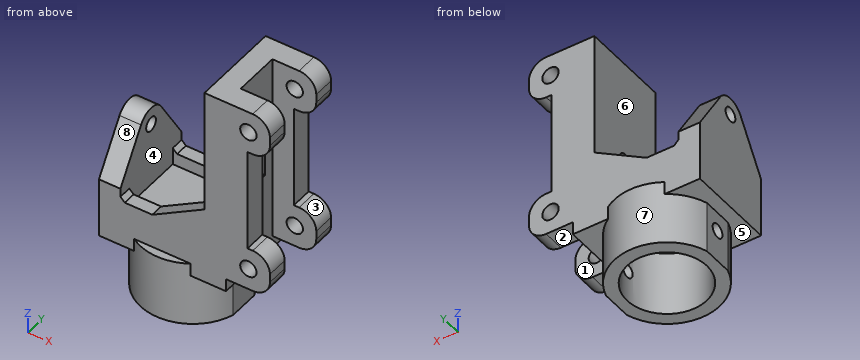
from build123d import *

# Parameters (mm, degrees)
SKETCH_1_R               = 6.325
EXTRUDE_1_DEPTH          = 15
SKETCH_2_W               = 29.5
SKETCH_2_H               = 20.7
EXTRUDE_2_DEPTH          = 5
SKETCH_3_W               = 39
SKETCH_3_H               = 20.7
SKETCH_3_R               = 1.65
EXTRUDE_3_DEPTH          = 5
SKETCH_4_W               = 10
SKETCH_4_H               = 5
EXTRUDE_4_DEPTH          = 10.2
SKETCH_5_R               = 1.9
CUT_EXTRUDE_1_DEPTH      = 21.7
FILLET_1_R               = 4
SKETCH_8_W               = 24
SKETCH_8_H               = 5
EXTRUDE_6_DEPTH          = 5
SKETCH_9_R               = 1.65
EXTRUDE_7_DEPTH          = 5
EXTRUDE_5_DEPTH          = 3
CHAMFER_2_SIZE           = 1
SKETCH_10_W              = 6.3
SKETCH_10_H              = 5.8
CUT_EXTRUDE_2_DEPTH      = 2.5
SKETCH_11_R              = 1.65
CUT_EXTRUDE_3_DEPTH      = 25.95
CUT_EXTRUDE_3_DEPTH_BACK = 15.75
CHAMFER_3_SIZE           = 1
CUT_EXTRUDE_4_DEPTH      = 1
CUT_EXTRUDE_4_DEPTH_BACK = 21.7
SKETCH_13_R              = 12.25
SKETCH_13_R_2            = 9.25
EXTRUDE_8_DEPTH          = 15
SKETCH_14_R              = 1.65
CUT_EXTRUDE_5_DEPTH      = 25.95
CUT_EXTRUDE_5_DEPTH_BACK = 15.75
SKETCH_15_W              = 4.137033229
SKETCH_15_H              = 7
CUT_EXTRUDE_6_DEPTH      = 15
EXTRUDE_9_DEPTH          = 3


with BuildPart() as part:
    # ｽｹｯﾁ1 → ﾎﾞｽ - 押し出し1 (new body)
    with BuildSketch(Plane.XY):
        Circle(SKETCH_1_R)
    extrude(amount=-EXTRUDE_1_DEPTH)

    # ｽｹｯﾁ2 → ﾎﾞｽ - 押し出し2 (add)
    with BuildSketch(Plane.XY):
        Rectangle(SKETCH_2_W, SKETCH_2_H)
    extrude(amount=EXTRUDE_2_DEPTH)

    # ｽｹｯﾁ3 → ﾎﾞｽ - 押し出し3 (add)
    with BuildSketch(Plane(origin=(14.75, 0, 0), x_dir=(0, 0, -1), z_dir=(1, 0, 0))):
        with Locations((-24.5, 0)):
            Rectangle(SKETCH_3_W, SKETCH_3_H)
        with Locations((-20, 0)):
            Circle(SKETCH_3_R, mode=Mode.SUBTRACT)
    extrude(amount=-EXTRUDE_3_DEPTH)

    # ｽｹｯﾁ4 → ﾎﾞｽ - 押し出し4 (add)
    with BuildSketch(Plane(origin=(14.75, 0, 0), x_dir=(0, 0, -1), z_dir=(1, 0, 0))):
        with Locations((-5, 7.85)):
            Rectangle(SKETCH_4_W, SKETCH_4_H)
        with Locations((-5, -7.85)):
            Rectangle(SKETCH_4_W, SKETCH_4_H)
        with Locations((-39, 7.85)):
            Rectangle(SKETCH_4_W, SKETCH_4_H)
        with Locations((-39, -7.85)):
            Rectangle(SKETCH_4_W, SKETCH_4_H)
    extrude(amount=EXTRUDE_4_DEPTH)

    # ｽｹｯﾁ5 → ｶｯﾄ - 押し出し1 (cut, through all)
    with BuildSketch(Plane.XZ.offset(10.35)):
        with Locations((19.95, 5)):
            Circle(SKETCH_5_R)
        with Locations((19.95, 39)):
            Circle(SKETCH_5_R)
    extrude(amount=-CUT_EXTRUDE_1_DEPTH, mode=Mode.SUBTRACT)

    # ﾌｨﾚｯﾄ1
    fillet_1_edges = [part.edges().sort_by_distance(p)[0] for p in [
        (24.95, 7.85, 0),
        (24.95, 7.85, 10),
        (24.95, -7.85, 0),
        (24.95, -7.85, 10),
        (24.95, -7.85, 44),
        (24.95, -7.85, 34),
        (24.95, 7.85, 44),
        (24.95, 7.85, 34),
    ]]
    fillet(fillet_1_edges, radius=FILLET_1_R)

    # ｽｹｯﾁ8 → ﾎﾞｽ - 押し出し6 (add)
    with BuildSketch(Plane(origin=(14.75, 0, 0), x_dir=(0, 0, -1), z_dir=(1, 0, 0))):
        with Locations((-22, 7.85)):
            Rectangle(SKETCH_8_W, SKETCH_8_H)
        with Locations((-22, -7.85)):
            Rectangle(SKETCH_8_W, SKETCH_8_H)
    extrude(amount=EXTRUDE_6_DEPTH)

    # ｽｹｯﾁ9 → ﾎﾞｽ - 押し出し7 (add)
    with BuildSketch(Plane.ZY.offset(14.75)):
        with BuildLine():
            Line((5, 10.35), (11, 10.35))
            Line((11, 10.35), (22.121751649, 3.390895153))
            ThreePointArc((22.121751649, 3.390895153), (24, 0), (22.121751649, -3.390895153))
            Line((22.121751649, -3.390895153), (11, -10.35))
            Line((11, -10.35), (5, -10.35))
            Line((5, -10.35), (5, 10.35))
        make_face()
        with Locations((20, 0)):
            Circle(SKETCH_9_R, mode=Mode.SUBTRACT)
    extrude(amount=-EXTRUDE_7_DEPTH)

    # ｽｹｯﾁ6 → ﾎﾞｽ - 押し出し5 (add)
    with BuildSketch(Plane.XZ.offset(10.35)):
        Polygon((-9.75, 5), (9.75, 5), (9.75, 15), (-2.374355653, 8), (-9.75, 8), align=None)
    extrude_5 = extrude(amount=-EXTRUDE_5_DEPTH)

    # ﾐﾗｰ1: ﾎﾞｽ - 押し出し5 across plane
    add(extrude_5.mirror(Plane.ZX))

    # 面取り2
    chamfer_2_edges = [part.edges().sort_by_distance(p)[0] for p in [
        (-9.75, -8.85, 8),
        (-9.75, 8.85, 8),
    ]]
    chamfer(chamfer_2_edges, length=CHAMFER_2_SIZE)

    # ｽｹｯﾁ10 → ｶｯﾄ - 押し出し2 (cut)
    with BuildSketch(Plane(origin=(14.75, 0, 0), x_dir=(0, 0, -1), z_dir=(1, 0, 0))):
        with Locations((-20, 0)):
            Rectangle(SKETCH_10_W, SKETCH_10_H)
    extrude(amount=-CUT_EXTRUDE_2_DEPTH, mode=Mode.SUBTRACT)

    # ｽｹｯﾁ11 → ｶｯﾄ - 押し出し3 (cut, two sides)
    with BuildSketch(Plane(origin=(0, 0, 0), x_dir=(0, 0, -1), z_dir=(1, 0, 0))) as cut_extrude_3_sk:
        with Locations((7.5, 0)):
            Circle(SKETCH_11_R)
    extrude(amount=CUT_EXTRUDE_3_DEPTH, mode=Mode.SUBTRACT)
    extrude(cut_extrude_3_sk.sketch, amount=-CUT_EXTRUDE_3_DEPTH_BACK, mode=Mode.SUBTRACT)

    # 面取り3
    chamfer_3_edges = [part.edges().sort_by_distance(p)[0] for p in [
        (-6.325, 0, -15),
    ]]
    chamfer(chamfer_3_edges, length=CHAMFER_3_SIZE)

    # ｽｹｯﾁ12 → ｶｯﾄ - 押し出し4 (cut, two sides)
    with BuildSketch(Plane(origin=(0, 10.35, 0), x_dir=(1, 0, 0), z_dir=(0, 1, 0))) as cut_extrude_4_sk:
        Polygon((-157.887970151, 0), (-20.856584832, 0), (30.621949215, 0), (167.653334534, 0), (167.653334534, 274.062770638), (-157.887970151, 274.062770638), align=None)
    extrude(amount=CUT_EXTRUDE_4_DEPTH, mode=Mode.SUBTRACT)
    extrude(cut_extrude_4_sk.sketch, amount=-CUT_EXTRUDE_4_DEPTH_BACK, mode=Mode.SUBTRACT)

    # ｽｹｯﾁ13 → ﾎﾞｽ - 押し出し8 (add)
    with BuildSketch(Plane(origin=(0, 0, 0), x_dir=(-1, 0, 0), z_dir=(0, 0, -1))):
        Circle(SKETCH_13_R)
        Circle(SKETCH_13_R_2, mode=Mode.SUBTRACT)
    extrude(amount=EXTRUDE_8_DEPTH)

    # ｽｹｯﾁ14 → ｶｯﾄ - 押し出し5 (cut, two sides)
    with BuildSketch(Plane(origin=(0, 0, 0), x_dir=(0, 0, -1), z_dir=(1, 0, 0))) as cut_extrude_5_sk:
        with Locations((7.5, 0)):
            Circle(SKETCH_14_R)
    extrude(amount=CUT_EXTRUDE_5_DEPTH, mode=Mode.SUBTRACT)
    extrude(cut_extrude_5_sk.sketch, amount=-CUT_EXTRUDE_5_DEPTH_BACK, mode=Mode.SUBTRACT)

    # ｽｹｯﾁ15 → ｶｯﾄ - 押し出し6 (cut)
    with BuildSketch(Plane(origin=(0, 0, -15), x_dir=(-1, 0, 0), z_dir=(0, 0, -1))):
        with Locations((-13.807873497, 0)):
            Rectangle(SKETCH_15_W, SKETCH_15_H)
        with Locations((13.807873497, 0)):
            Rectangle(SKETCH_15_W, SKETCH_15_H)
    extrude(amount=-CUT_EXTRUDE_6_DEPTH, mode=Mode.SUBTRACT)

    # ｽｹｯﾁ16 → ﾎﾞｽ - 押し出し9 (add)
    with BuildSketch(Plane(origin=(0, 0, 0), x_dir=(-1, 0, 0), z_dir=(0, 0, -1))):
        with BuildLine():
            Line((-11.739356882, 3.5), (-11.739356882, -3.5))
            ThreePointArc((-11.739356882, -3.5), (-9.766367935, -7.394630306), (-6.55286197, -10.35))
            Line((-6.55286197, -10.35), (-14.75, -10.35))
            Line((-14.75, -10.35), (-14.75, 10.35))
            Line((-14.75, 10.35), (-6.55286197, 10.35))
            ThreePointArc((-6.55286197, 10.35), (-9.766367935, 7.394630306), (-11.739356882, 3.5))
        make_face()
        with BuildLine():
            Line((6.55286197, -10.35), (14.75, -10.35))
            Line((14.75, -10.35), (14.75, 10.35))
            Line((14.75, 10.35), (6.55286197, 10.35))
            ThreePointArc((6.55286197, 10.35), (9.766367935, 7.394630306), (11.739356882, 3.5))
            Line((11.739356882, 3.5), (11.739356882, -3.5))
            ThreePointArc((11.739356882, -3.5), (9.766367935, -7.394630306), (6.55286197, -10.35))
        make_face()
    extrude(amount=EXTRUDE_9_DEPTH)


solid = part.part
Build history of the part. All positions in model axes, mm. Face numbers are marked on the shaded views. A direction names the side the tool comes from. Round coordinates to 2 decimals unless told otherwise and drop trailing zeros. Write each loop counter-clockwise with the first axis right and the second up, starting at its lowest first coordinate (ties: lowest second). Pieces come first, ordered by that corner, then holes. Notation, with made-up numbers: (56, 86.25) - (78, 86.25) arc R22 ccw to (78, 124.25) - close; hole circle Ø2 at (41, 81). An arc over 180 degrees is marked (long way). Use CSV: the item, a comma, the result in double quotes.
(1) Wall check: line 1 (Z direction, x = 19.95, y = -8.15); line 2 (Z direction, x = 19, y = -5.5); line 3 (Y direction, x = 10, z = 20). Give the ranges that are in metal, low to high.
Response:
line 1,"0 to 3.1, 6.9 to 10, 34 to 37.1, 40.9 to 44"
line 2,"0 to 3.35, 6.65 to 37.35, 40.65 to 44"
line 3,"-10.35 to -1.65, 1.65 to 10.35"
(2) Mould opens along X. For the marked faces 6, 7 and 8 say: pulls with the +X half, pulls with the -X half, needs draft (parallel to the pull), parting line crosses it, or undercut.
Response:
face 6,"undercut"
face 7,"parting line crosses it"
face 8,"needs draft"
(3) Pin check, flat tips, straight feed: P1, Ø1.5, axis at x = 19, z = 21, coming from the +Y side; P2, Ø2.5, axis at y = 0, z = 20, coming from the +X side; P3, Ø6, axis at x = 11, z = 9.5, coming from the -Y side; P4, Ø1.5, axis at y = -7.5, z = 11, coming from the +X side. Stop position of each tip, or through.
Response:
P1,"y = 10.35"
P2,"through"
P3,"y = -10.35"
P4,"x = 19.75"
(4) Band-saw the part on A-A (z = 39). Write the cut outline in (x, y), plus the area to 4 significant figures.
Response:
outline,"(9.75, -10.35) - (18.05, -10.35) - (18.05, -5.35) - (14.75, -5.35) - (14.75, 5.35) - (18.05, 5.35) - (18.05, 10.35) - (9.75, 10.35) - close; (21.85, -10.35) - (24.95, -10.35) - (24.95, -5.35) - (21.85, -5.35) - close; (21.85, 5.35) - (24.95, 5.35) - (24.95, 10.35) - (21.85, 10.35) - close"
area,"167.5 mm²"
(5) Band-saw the part on D-D (x = 0). Write the cut outline in (y, z), plus the area to 3 significant figures.
Response:
outline,"(-12.25, -15) - (-9.25, -15) - (-9.25, 0) - (9.25, 0) - (9.25, -15) - (12.25, -15) - (12.25, 0) - (10.35, 0) - (10.35, 9.37) - (7.35, 9.37) - (7.35, 5) - (-7.35, 5) - (-7.35, 9.37) - (-10.35, 9.37) - (-10.35, 0) - (-12.25, 0) - close"
area,"220 mm²"
(6) Band-saw the part on C-C (z = 20). Write the cut outline in (x, y), plus the area to 3 significant figures.
Response:
outline,"(-14.75, -4.72) - (-9.75, -4.72) - (-9.75, -1.65) - (-14.75, -1.65) - close; (-14.75, 1.65) - (-9.75, 1.65) - (-9.75, 4.72) - (-14.75, 4.72) - close; (9.75, -10.35) - (19.75, -10.35) - (19.75, -5.35) - (14.75, -5.35) - (14.75, -2.9) - (12.25, -2.9) - (12.25, -1.65) - (9.75, -1.65) - close; (9.75, 1.65) - (12.25, 1.65) - (12.25, 2.9) - (14.75, 2.9) - (14.75, 5.35) - (19.75, 5.35) - (19.75, 10.35) - (9.75, 10.35) - close"
area,"161 mm²"
(7) Band-saw the part on B-B (z = 33). Write the cut outline in (x, y), plus the area to 4 significant figures.
Response:
outline,"(9.75, -10.35) - (19.75, -10.35) - (19.75, -5.35) - (14.75, -5.35) - (14.75, 5.35) - (19.75, 5.35) - (19.75, 10.35) - (9.75, 10.35) - close"
area,"153.5 mm²"
(8) 3-axis set-ups, long thin cutter, end or side, ignore diameter. For the marked faces 1, 2, 3, 4 and 5: which of +Z, -Z, +X, -X, +Y, -Y reach the whole face in a straight line?
Response:
face 1,"+Z, -Z, +X"
face 2,"-Z, +X, +Y, -Y"
face 3,"+X, +Y, -Y"
face 4,"+Z"
face 5,"-Z, -X"
